The model under review builds one solid part; all positions refer to its coordinate system, in mm. A direction names the side the tool comes from. Give positions to 0.01 mm unless a question says otherwise; leave off trailing zeros. Order: outer loops, then holes, each group sorted by start corner. A loop starts at its lowest first (then second) coordinate and runs counter-clockwise, first axis right, second up.
Autodesk Inventor part; units mm, degrees
ref_plane "YZ Plane" through (0, 0, 0) normal (1, 0, 0) x (0, 1, 0)
ref_plane "XZ Plane" through (0, 0, 0) normal (0, 1, 0) x (-1, 0, 0)
ref_plane "Work Plane1" through (0, 0, 200) normal (0, 0, 1) x (1, 0, 0)
sketch "Sketch1" plane through (0, 0, 200) normal (0, 0, 1) x (1, 0, 0)
  line L0 (0, 8.259) -> (0, -5.5938)
  line L1 (-6.2911, 0) -> (6.8799, 0)
  line L2 (0, 94) -> (-100, 94)
  line L3 (-100, 94) -> (-100, 29)
  line L4 (-100, 29) -> (-50, 29)
  line L5 (-50, 29) -> (-50, -35)
  line L6 (-50, -35) -> (0, -35)
  line L7 (0, 94) -> (100, 94)
  line L8 (100, 94) -> (100, 29)
  line L9 (100, 29) -> (50, 29)
  line L10 (50, 29) -> (50, -35)
  line L11 (50, -35) -> (0, -35)
  point P0 (0, 0)
  dimension "d1" = 100
  dimension "d2" = 188
  dimension "d3" = 65
  dimension "d5" = 50
  dimension "d21" = 64
extrude "Extrusion1" add sketch "Sketch1" along normal blind 150
sketch "Sketch2" plane through (0, 0, 200) normal (0, 0, 1) x (1, 0, 0)
  circle A0 centre (0, 0) radius 13
  dimension "d8" = 26
extrude "Extrusion2" add sketch "Sketch2" against normal blind 170
sketch "Sketch3" plane through (0, 0, 200) normal (0, 0, -1) x (-1, 0, 0)
  line L0 (20, -20) -> (-20, -20)
  line L1 (-20, -20) -> (-20, 20)
  line L2 (-20, 20) -> (20, 20)
  line L3 (20, 20) -> (20, -20)
  line L4 (0, -60.8) -> (0, 119.8)
  line L5 (140, 0) -> (-140, 0)
  point P0 (0, 0)
  dimension "d11" = 40
  dimension "d12" = 40
extrude "Extrusion3" add sketch "Sketch3" along normal blind 60
chamfer "Chamfer1" distance 5 angle 45 4 edges at (-20, -20, 170) (-20, 20, 170) (20, -20, 170) (20, 20, 170)
chamfer "Chamfer2" distance 2 angle 45 1 edges at (-13, 0, 30)
sketch "Sketch4" plane through (0, 0, 350) normal (0, 0, 1) x (1, 0, 0)
  line L0 (0, -53.3893) -> (0, 113.7531)
  line L1 (100, 94) -> (-100, 94)
  line L2 (82, 94) -> (62, 94)
  line L3 (62, 94) -> (62, 78)
  line L4 (62, 78) -> (82, 78)
  line L5 (82, 78) -> (82, 94)
  line L6 (100, 29) -> (100, 94)
  line L7 (-82, 94) -> (-62, 94)
  line L8 (-62, 94) -> (-62, 78)
  line L9 (-62, 78) -> (-82, 78)
  line L10 (-82, 78) -> (-82, 94)
  point P0 (0, 0)
  dimension "d22" = 20
  dimension "d23" = 16
  dimension "d24" = 18
extrude "Extrusion4" cut sketch "Sketch4" against normal through all
properties part number "Z_axis"
Item 1: Clearance check with flat-ended pins moving along their axes: pin 1 Ø15 at (x, z) = (84, 295.5) entering from -Y; pin 2 Ø1.5 at (x, y) = (-14, 18.5) entering from -Z; pin 3 Ø24 at (x, z) = (6.5, 172.5) entering from -Y. State where each tip first meets the part, or that it passes through.
Values found:
pin 1: stops at y = 29
pin 2: stops at z = 140
pin 3: stops at y = -20
Item 2: For line 1 (Z direction, x = -46.5, y = -22.5); line 2 (X direction, y = 2.5, z = 257.5); line 3 (Y direction, x = 57.5, z = 218.5), list the stretches that pass through material, from the lowest coordinate up.
Values found:
line 1: z = 200 to 350
line 2: x = -50 to 50
line 3: y = 29 to 94
Item 3: Take a section at D-D (y = -27). Give the boundary of the cut face in (x, z).
Values found:
outline: (-50, 200) - (50, 200) - (50, 350) - (-50, 350) - close
Item 4: For faces 1 (the flat face through (50, -3, 274)), 2 (the flat face through (-50, -3, 274)), 3 (the flat face through (0, 20, 170)), list the 3-axis set-ups (+Z, -Z, +X, -X, +Y, -Y) from which the entire face can be reached by the end or side of a thin tool; tool diameter is ignored.
Values found:
face 1: +Z, -Z, +X, -Y
face 2: +Z, -Z, -X, -Y
face 3: -Z, +X, -X, +Y
Item 5: Take a section at A-A (y = 81.5). Give the boundary of the cut face in (x, z).
Values found:
outline: (-100, 200) - (-82, 200) - (-82, 350) - (-100, 350) - close; (-62, 200) - (62, 200) - (62, 350) - (-62, 350) - close; (82, 200) - (100, 200) - (100, 350) - (82, 350) - close
Item 6: Take a section at B-B (x = 0). Give the boundary of the cut face in (y, z).
Values found:
outline: (-35, 200) - (-20, 200) - (-20, 140) - (-13, 140) - (-13, 32) - (-11, 30) - (11, 30) - (13, 32) - (13, 140) - (20, 140) - (20, 200) - (94, 200) - (94, 350) - (-35, 350) - close
Item 7: Take a section at C-C (z = 246). Give the boundary of the cut face in (x, y).
Values found:
outline: (-100, 29) - (-50, 29) - (-50, -35) - (50, -35) - (50, 29) - (100, 29) - (100, 94) - (82, 94) - (82, 78) - (62, 78) - (62, 94) - (-62, 94) - (-62, 78) - (-82, 78) - (-82, 94) - (-100, 94) - close
